```python
from build123d import *

# Parameters (mm, degrees)
BOSS_EXTRUDE2_DEPTH = 10
SKETCH2_W           = 10
SKETCH2_H           = 10
BOSS_EXTRUDE3_DEPTH = 5


with BuildPart() as part:
    # Sketch1 → Boss-Extrude2 (new body)
    with BuildSketch(Plane.XY):
        with BuildLine():
            ThreePointArc((0, 60), (17.573593129, 17.573593129), (60, 0))
            ThreePointArc((60, 0), (17.573593129, -17.573593129), (0, -60))
            ThreePointArc((0, -60), (-17.573593129, -17.573593129), (-60, 0))
            ThreePointArc((-60, 0), (-17.573593129, 17.573593129), (0, 60))
        make_face()
    extrude(amount=BOSS_EXTRUDE2_DEPTH)

    # Sketch2 → Boss-Extrude3 (add, symmetric)
    with BuildSketch(Plane.XY.offset(10)):
        with Locations((-0.141365773, -60.179831665)):
            Rectangle(SKETCH2_W, SKETCH2_H)
        with Locations((59.60084876, -0.244611601)):
            Rectangle(SKETCH2_W, SKETCH2_H)
        with Locations((-59.798330542, 0.00957883)):
            Rectangle(SKETCH2_W, SKETCH2_H)
        with Locations((-0.007106667, 59.651317451)):
            Rectangle(SKETCH2_W, SKETCH2_H)
    extrude(amount=BOSS_EXTRUDE3_DEPTH, both=True)


solid = part.part
```
Geometry: final body of the model. Coordinates: model frame, mm. A direction names the side the tool comes from. Give positions to 0.01 mm unless a question says otherwise; leave off trailing zeros. Write each loop counter-clockwise with the first axis right and the second up, starting at its lowest first coordinate (ties: lowest second). Pieces come first, ordered by that corner, then holes.
1. Line query: probe 1 along Y at (x, z) = (59.5, 11); probe 2 along Z at (x, y) = (0, -3); probe 3 along Y at (x, z) = (9, 1.25). Output: solid intervals per line, ascending.
2. Section query D-D, the plane x = 20. Return loops of the section in (y, z), then the cut area to 3 significant figures.
3. Pin query (flat end, axial travel): P1, Ø5, axis at x = -59.5, z = 8.5, coming from the +Y side; P2, Ø8, axis at y = 58.5, z = 10.5, coming from the -X side; P3, Ø1.5, axis at x = 8.5, z = 7, coming from the -Y side. Return the tip coordinate at first contact, or that it passes through.
4. Reachability of faces 1 (the flat face through (4.993, 60, 10)), 2 (the flat face through (-61, 0, 5)), 3 (the flat face through (4.859, -60, 10)), 4 (the flat face through (-60, 5.01, 10)) from +Z, -Z, +X, -X, +Y, -Y: full face, straight path, thin tool, end or side. Return the list, or none.
5. Draft query along X for faces 5 (the flat face through (60, -5.245, 10)), 6 (the flat face through (64.601, 0, 10)), 7 (the flat face through (-54.798, 0, 11)). Return one class per face: released by +X, released by -X, zero draft, split by the parting line, or undercut.
6. Section query C-C, the plane z = 6.5. Return loops of the section in (x, y), then the cut area to 3 significant figures.
7. Section query A-A, the plane z = 13.5. Return loops of the section in (x, y), then the cut area to 3 significant figures.
8. Section query B-B, the plane y = 57.5. Return loops of the section in (x, z).
Computed:
1. probe 1: y = -5.24 to 4.76
1. probe 2: z = 0 to 10
1. probe 3: y = -28.39 to 28.39
2. outline: (-15.28, 0) - (15.28, 0) - (15.28, 10) - (-15.28, 10) - close
2. area: 306 mm2
3. P1: stops at y = 5.01
3. P2: stops at x = -5.01
3. P3: stops at y = -30.51
4. face 1: +Z, -Z, +X, +Y
4. face 2: -Z, -X
4. face 3: +Z, -Z, +X, -Y
4. face 4: +Z, -Z, -X, +Y
5. face 5: zero draft
5. face 6: released by +X
5. face 7: undercut
6. outline: (-64.8, -4.99) - (-54.8, -4.99) - (-54.8, -0.23) arc R60 cw to (-0.19, -55.18) - (-5.14, -55.18) - (-5.14, -65.18) - (4.86, -65.18) - (4.86, -55.18) - (0.19, -55.18) arc R60 cw to (54.6, -0.24) - (54.6, -5.24) - (64.6, -5.24) - (64.6, 4.76) - (54.6, 4.76) - (54.6, 0.24) arc R60 cw to (0.24, 54.65) - (4.99, 54.65) - (4.99, 64.65) - (-5.01, 64.65) - (-5.01, 54.65) - (-0.24, 54.65) arc R60 cw to (-54.8, 0.23) - (-54.8, 5.01) - (-64.8, 5.01) - close
6. area: 3,490 mm2
7. outline: (-64.8, -4.99) - (-54.8, -4.99) - (-54.8, 5.01) - (-64.8, 5.01) - close; (-5.14, -65.18) - (4.86, -65.18) - (4.86, -55.18) - (-5.14, -55.18) - close; (-5.01, 54.65) - (4.99, 54.65) - (4.99, 64.65) - (-5.01, 64.65) - close; (54.6, -5.24) - (64.6, -5.24) - (64.6, 4.76) - (54.6, 4.76) - close
7. area: 400 mm2
8. outline: (-5.01, 5) - (-0.05, 5) - (-0.05, 0) - (0.05, 0) - (0.05, 5) - (4.99, 5) - (4.99, 15) - (-5.01, 15) - close
